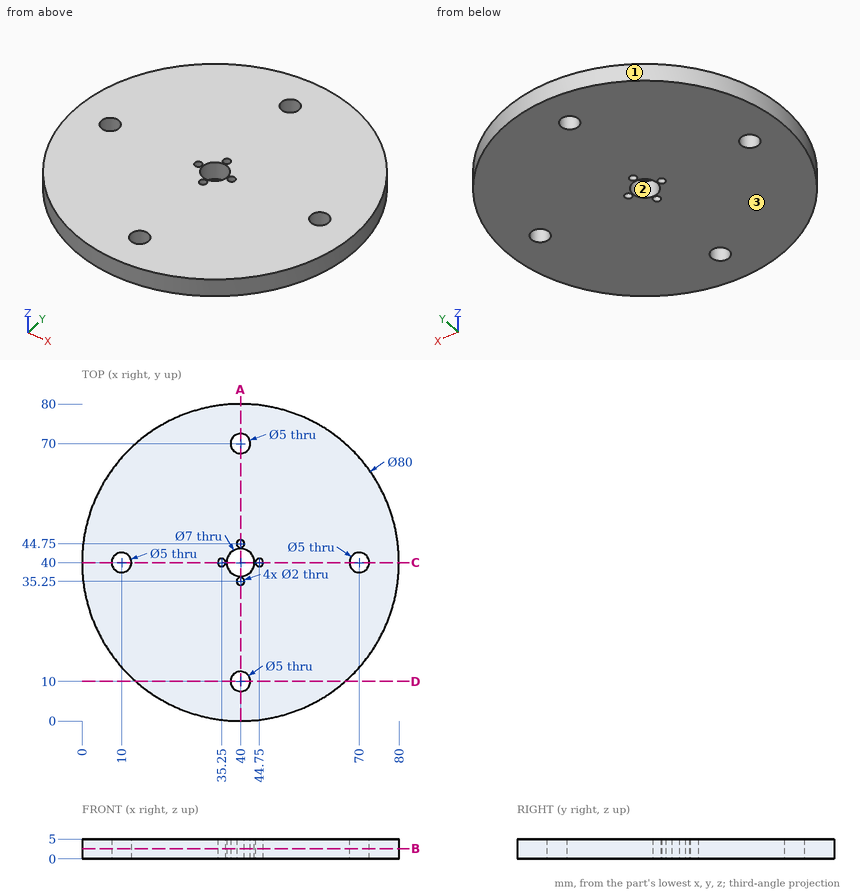
Could you check a few things on this drawing? It's one solid part, dimensions in mm from its lowest x, y, z. Round coordinates to 2 decimals unless told otherwise and drop trailing zeros. Write each loop counter-clockwise with the first axis right and the second up, starting at its lowest first coordinate (ties: lowest second). Pieces come first, ordered by that corner, then holes. Notation, with made-up numbers: (59, 33) -> (116, 33) arc R21 cw to (116, 49) -> close; hole circle Ø7 at (-37, 87.25). An arc over 180 degrees is marked (long way). Use one line per item in the form item = value. Start each with the question number.
Q1. I'm going to push flat-ended pins straight in: P1, Ø1, axis at y = 53.5, z = 4.5, coming from the +X side; P2, Ø4, axis at x = 40, y = 40, coming from the -Z side. Where does each tip first touch, or does it pass through?
Q2. Imagine slicing it at B-B (z = 2.6). Count the separate pieces of the cut face and the enclosed holes in it, then the cut area to 3 significant figures.
Q3. If I drill on probe 1 along Y at (x, z) = (40, 3); probe 2 along X at (y, z) = (10.5, 0.85); probe 3 along X at (y, z) = (70, 3.7), over which ranges is the centre line in solid material (lowest first)? Write a range as [from, to].
Q4. Imagine slicing it at D-D (y = 10). Please give me the cut outline in (x, z), then the cut area to 3 significant figures.
Q5. We'd pull the mould along X, two halves only. Please class the marked faces 1, 2 and 3: +X half, -X half, draft (parallel to the pull), parting line (faces both ways), or undercut.
Q6. Imagine slicing it at A-A (x = 40). Please give me the cut outline in (y, z), then the cut area to 3 significant figures.
Worked out:
q1.P1 = 77.83
q1.P2 = through
q2.separate_pieces = 1
q2.enclosed_holes = 9
q2.area = 4,900 mm^2
q3.probe_1 = [0, 7.5], [12.5, 34.25], [36.25, 36.5], [43.5, 43.75], [45.75, 67.5], [72.5, 80]
q3.probe_2 = [12.99, 37.55], [42.45, 67.01]
q3.probe_3 = [13.54, 37.5], [42.5, 66.46]
q4.outline = (13.54, 0) -> (37.5, 0) -> (37.5, 5) -> (13.54, 5) -> close; (42.5, 0) -> (66.46, 0) -> (66.46, 5) -> (42.5, 5) -> close
q4.area = 240 mm^2
q5.face_1 = parting line
q5.face_2 = undercut
q5.face_3 = draft
q6.outline = (0, 0) -> (7.5, 0) -> (7.5, 5) -> (0, 5) -> close; (12.5, 0) -> (34.25, 0) -> (34.25, 5) -> (12.5, 5) -> close; (36.25, 0) -> (36.5, 0) -> (36.5, 5) -> (36.25, 5) -> close; (43.5, 0) -> (43.75, 0) -> (43.75, 5) -> (43.5, 5) -> close; (45.75, 0) -> (67.5, 0) -> (67.5, 5) -> (45.75, 5) -> close; (72.5, 0) -> (80, 0) -> (80, 5) -> (72.5, 5) -> close
q6.area = 295 mm^2
